from build123d import *

# Parameters (mm, degrees)
SKETCH4_W           = 50
SKETCH4_H           = 50
BOSS_EXTRUDE2_DEPTH = 2
CUT_EXTRUDE1_REACH  = 72.739
SKETCH5_R           = 0.825
CUT_EXTRUDE2_REACH  = 72.739
SKETCH6_R           = 3.525


with BuildPart() as part:
    # Sketch4 → Boss-Extrude2 (new body)
    with BuildSketch(Plane.XY):
        with Locations((-25, 25)):
            Rectangle(SKETCH4_W, SKETCH4_H)
    extrude(amount=BOSS_EXTRUDE2_DEPTH)

    # Sketch5 → Cut-Extrude1 (cut, up to next)
    with BuildSketch(Plane.XY.offset(2), mode=Mode.PRIVATE) as cut_extrude1_sk1:
        with Locations((-25, 30.5)):
            Circle(SKETCH5_R)
    cut_extrude1_tool1 = extrude(cut_extrude1_sk1.sketch, amount=-CUT_EXTRUDE1_REACH, mode=Mode.PRIVATE) & part.part
    # Sketch5 → Cut-Extrude1 (cut, up to next)
    with BuildSketch(Plane.XY.offset(2), mode=Mode.PRIVATE) as cut_extrude1_sk2:
        with Locations((-25, 19.5)):
            Circle(SKETCH5_R)
    cut_extrude1_tool2 = extrude(cut_extrude1_sk2.sketch, amount=-CUT_EXTRUDE1_REACH, mode=Mode.PRIVATE) & part.part
    add(cut_extrude1_tool1.solids().sort_by_distance((-25, 30.5, 2))[0], mode=Mode.SUBTRACT)
    add(cut_extrude1_tool2.solids().sort_by_distance((-25, 19.5, 2))[0], mode=Mode.SUBTRACT)

    # Sketch6 → Cut-Extrude2 (cut, up to next)
    with BuildSketch(Plane(origin=(0, 0, 0), x_dir=(-1, 0, 0), z_dir=(0, 0, -1)), mode=Mode.PRIVATE) as cut_extrude2_sk1:
        with Locations((25, 25)):
            Circle(SKETCH6_R)
    cut_extrude2_tool1 = extrude(cut_extrude2_sk1.sketch, amount=-CUT_EXTRUDE2_REACH, mode=Mode.PRIVATE) & part.part
    add(cut_extrude2_tool1.solids().sort_by_distance((-25, 25, 0))[0], mode=Mode.SUBTRACT)


solid = part.part
Source: CAD feature listing. Evaluate the final solid. Frame: model axes, mm. Give positions to 0.01 mm unless a question says otherwise; leave off trailing zeros. Loops run counter-clockwise (first coordinate to the right, second up) from the corner with the lowest first, then second, coordinate; pieces in that order, holes last. Notation, with made-up numbers: (10.5, 5.5) -> (40.5, 5.5) arc R13 cw to (40.5, 28.5) -> close; hole circle Ø7 at (13.5, -39). An arc over 180 degrees is marked (long way). Use a Markdown table: item, result. Add a question column.
1) Section query A-A, the plane x = -25. Return the cut outline in (y, z) (3 decimals).
2) Line query: line 1 along Y through (x, z) = (-25, 0.95) (3 decimals); line 2 along X through (y, z) = (31, 0.95); line 3 along X through (y, z) = (23.5, 0.15). Output: solid intervals per line, ascending. Write a range as [from, to].
3) Section query D-D, the plane y = 26.5. Return the cut outline in (x, z), then the cut area to 3 significant figures.
4) First-contact query: pin 1 (2.5 mm diameter, centred on x = -25, y = 19.5, fed in from -Z). Flat tip, straight axial feed; report the tip coordinate or a pass-through.
5) Pull-direction query (X, two-part tool) for faces 1 (the face through (-31, 25, 2)), 2 (the face through (-25.2, 29.7, 1)), 3 (the face through (-50, 25, 1)); classes: +X half, -X half, draft (parallel to the pull), parting line (faces both ways), or undercut.
6) Section query C-C, the plane z = 1.1. Return the cut outline in (x, y) (3 decimals), then the cut area to 3 significant figures.
7) Section query B-B, the plane y = 19.5. Return the cut outline in (x, z) (3 decimals).
Numbers:
| question | item | result |
|---|---|---|
| 1 | outline | (0, 0) -> (18.675, 0) -> (18.675, 2) -> (0, 2) -> close; (20.325, 0) -> (21.475, 0) -> (21.475, 2) -> (20.325, 2) -> close; (28.525, 0) -> (29.675, 0) -> (29.675, 2) -> (28.525, 2) -> close; (31.325, 0) -> (50, 0) -> (50, 2) -> (31.325, 2) -> close |
| 2 | line 1 | y = [0, 18.675], [20.325, 21.475], [28.525, 29.675], [31.325, 50] |
| 2 | line 2 | x = [-50, -25.66], [-24.34, 0] |
| 2 | line 3 | x = [-50, -28.19], [-21.81, 0] |
| 3 | outline | (-50, 0) -> (-28.19, 0) -> (-28.19, 2) -> (-50, 2) -> close; (-21.81, 0) -> (0, 0) -> (0, 2) -> (-21.81, 2) -> close |
| 3 | area | 87.2 mm2 |
| 4 | pin 1 | stops at z = 0 |
| 5 | face 1 | draft |
| 5 | face 2 | undercut |
| 5 | face 3 | -X half |
| 6 | outline | (-50, 0) -> (0, 0) -> (0, 50) -> (-50, 50) -> close; hole circle Ø7.05 at (-25, 25); hole circle Ø1.65 at (-25, 19.5); hole circle Ø1.65 at (-25, 30.5) |
| 6 | area | 2,460 mm2 |
| 7 | outline | (-50, 0) -> (-25.825, 0) -> (-25.825, 2) -> (-50, 2) -> close; (-24.175, 0) -> (0, 0) -> (0, 2) -> (-24.175, 2) -> close |
